Input: part model. Units: mm. Frame: model coordinates. Round coordinates to 2 decimals unless told otherwise and drop trailing zeros. One line per question, with ' | ' between items. Start each with the question number.
from build123d import *

# Parameters (mm, degrees)
CROQUIS1_R              = 2.5
SALIENTE_EXTRUIR1_DEPTH = 5
REDONDEO1_R             = 5


with BuildPart() as part:
    # Croquis1 → Saliente-Extruir1 (new, symmetric)
    with BuildSketch(Plane(origin=(0, 0, 0), x_dir=(-1, 0, 0), z_dir=(0, 1, 0))):
        with BuildLine():
            Line((0, 7.5), (105, 7.5))
            ThreePointArc((105, 7.5), (112.5, 0), (105, -7.5))
            Line((105, -7.5), (0, -7.5))
            ThreePointArc((0, -7.5), (-7.5, 0), (0, 7.5))
        make_face()
        with Locations(Location((0, 0, 0), (0, 0, 90))):
            Circle(CROQUIS1_R, mode=Mode.SUBTRACT)
        with Locations(Location((105, 0, 0), (0, 0, 90))):
            Circle(CROQUIS1_R, mode=Mode.SUBTRACT)
    extrude(amount=SALIENTE_EXTRUIR1_DEPTH, both=True)

    # Redondeo1
    redondeo1_edges = [part.edges().sort_by_distance(p)[0] for p in [
        (7.5, 5, 0),
        (-52.5, 5, 7.5),
        (-112.5, 5, 0),
        (7.5, -5, 0),
        (-52.5, -5, 7.5),
        (-112.5, -5, 0),
        (-52.5, 5, -7.5),
        (-52.5, -5, -7.5),
    ]]
    fillet(redondeo1_edges, radius=REDONDEO1_R - 0.0001)  # a hair under: the kernel refuses the full size


solid = part.part
(1) Pull-direction query (Z, two-part tool) for faces 1 (the face through (-53, -5, 0)), 2 (the face through (-51.76, 3.57, -6)), 3 (the face through (-2.44, -0.07, -0.54)), 4 (the face through (-53.24, 3.57, 6)); classes: released by +Z, released by -Z, zero draft, split by the parting line, or undercut.
(2) Section B-B, the plane z = 0. Give the number of separate pieces and of enclosed holes in the cut face, plus the area to 3 significant figures.
(3) Line query: line 1 along X through (y, z) = (4, 0.75); line 2 along X through (y, z) = (2, 0); line 3 along Z through (x, y) = (-1.5, -0.5). Output: solid intervals per line, ascending. Write a range as from..to.
(4) Pin query (flat end, axial travel): P1, Ø4, axis at x = -105, z = 0, coming from the +Y side; P2, Ø5, axis at x = -24.5, z = 5.5, coming from the -Y side; P3, Ø1, axis at x = -10.5, z = -4, coming from the +Y side. Return the tip coordinate at first contact, or that it passes through.
Derived:
1) face 1: zero draft | face 2: released by -Z | face 3: undercut | face 4: released by +Z
2) separate pieces: 3 | enclosed holes: 0 | area: 1,080 mm²
3) line 1: x = -110.45..-107.38, -102.62..-2.38, 2.38..5.45 | line 2: x = -112.08..-107.5, -102.5..-2.5, 2.5..7.08 | line 3: z = -7.47..-2, 2..7.47
4) P1: passes through | P2: stops at y = -4.97 | P3: stops at y = 4.9
